Geometry: final body of the model. Coordinates: model frame, mm. A direction names the side the tool comes from. Give positions to 0.01 mm unless a question says otherwise; leave off trailing zeros. Order: outer loops, then holes, each group sorted by start corner. A loop starts at its lowest first (then second) coordinate and runs counter-clockwise, first axis right, second up. Notation, with made-up numbers: M 13,63.5 L 38,63.5 A30 ccw 38,91.5 Z; hole C 89.5,-5 d7. An arc over 180 degrees is marked long. Use CSV: the item, a comma, the result in double quotes.
```python
from build123d import *

# Parameters (mm, degrees)
BOSS_EXTRUDE2_DEPTH  = 4
SKETCH2_W            = 390
SKETCH2_H            = 480
BOSS_EXTRUDE3_DEPTH  = 4
SKETCH3_W            = 380
SKETCH3_H            = 470
BOSS_EXTRUDE4_DEPTH  = 4
SKETCH4_W            = 370
SKETCH4_H            = 460
BOSS_EXTRUDE5_DEPTH  = 4
SKETCH5_W            = 360
SKETCH5_H            = 450
BOSS_EXTRUDE6_DEPTH  = 4
SKETCH6_W            = 280
SKETCH6_H            = 370
CUT_EXTRUDE1_DEPTH   = 4
SKETCH7_W            = 270
SKETCH7_H            = 360
CUT_EXTRUDE2_DEPTH   = 4
SKETCH8_W            = 260
SKETCH8_H            = 350
CUT_EXTRUDE3_DEPTH   = 4
SKETCH9_W            = 250
SKETCH9_H            = 340
CUT_EXTRUDE4_DEPTH   = 4
SKETCH11_W           = 190
SKETCH11_H           = 280
BOSS_EXTRUDE7_DEPTH  = 4
SKETCH12_W           = 180
SKETCH12_H           = 270
BOSS_EXTRUDE8_DEPTH  = 4
SKETCH13_W           = 170
SKETCH13_H           = 260
BOSS_EXTRUDE9_DEPTH  = 4
SKETCH14_W           = 160
SKETCH14_H           = 250
BOSS_EXTRUDE10_DEPTH = 4
SKETCH15_W           = 20
SKETCH15_H           = 20
BOSS_EXTRUDE11_DEPTH = 5
SKETCH16_W           = 15
SKETCH16_H           = 15
BOSS_EXTRUDE12_DEPTH = 5
SKETCH17_W           = 10
SKETCH17_H           = 10
BOSS_EXTRUDE13_DEPTH = 20
BOSS_EXTRUDE14_REACH = 302
SKETCH18_W           = 10
SKETCH18_H           = 10
SKETCH19_W           = 35
SKETCH19_H           = 50
CUT_EXTRUDE5_DEPTH   = 3


with BuildPart() as part:
    # Sketch1 → Boss-Extrude2 (new body)
    with BuildSketch(Plane.XY):
        Polygon((200, 0), (200, -20), (200, -245), (-200, -245), (-200, -20), (-200, 0), (-200, 245), (200, 245), align=None)
    extrude(amount=BOSS_EXTRUDE2_DEPTH)

    # Sketch2 → Boss-Extrude3 (add)
    with BuildSketch(Plane.XY.offset(4)):
        Rectangle(SKETCH2_W, SKETCH2_H)
    extrude(amount=BOSS_EXTRUDE3_DEPTH)

    # Sketch3 → Boss-Extrude4 (add)
    with BuildSketch(Plane.XY.offset(8)):
        Rectangle(SKETCH3_W, SKETCH3_H)
    extrude(amount=BOSS_EXTRUDE4_DEPTH)

    # Sketch4 → Boss-Extrude5 (add)
    with BuildSketch(Plane.XY.offset(12)):
        Rectangle(SKETCH4_W, SKETCH4_H)
    extrude(amount=BOSS_EXTRUDE5_DEPTH)

    # Sketch5 → Boss-Extrude6 (add)
    with BuildSketch(Plane.XY.offset(16)):
        Rectangle(SKETCH5_W, SKETCH5_H)
    extrude(amount=BOSS_EXTRUDE6_DEPTH)

    # Sketch6 → Cut-Extrude1 (cut)
    with BuildSketch(Plane.XY.offset(20)):
        Rectangle(SKETCH6_W, SKETCH6_H)
    extrude(amount=-CUT_EXTRUDE1_DEPTH, mode=Mode.SUBTRACT)

    # Sketch7 → Cut-Extrude2 (cut)
    with BuildSketch(Plane.XY.offset(16)):
        Rectangle(SKETCH7_W, SKETCH7_H)
    extrude(amount=-CUT_EXTRUDE2_DEPTH, mode=Mode.SUBTRACT)

    # Sketch8 → Cut-Extrude3 (cut)
    with BuildSketch(Plane.XY.offset(12)):
        Rectangle(SKETCH8_W, SKETCH8_H)
    extrude(amount=-CUT_EXTRUDE3_DEPTH, mode=Mode.SUBTRACT)

    # Sketch9 → Cut-Extrude4 (cut)
    with BuildSketch(Plane.XY.offset(8)):
        Rectangle(SKETCH9_W, SKETCH9_H)
    extrude(amount=-CUT_EXTRUDE4_DEPTH, mode=Mode.SUBTRACT)

    # Sketch11 → Boss-Extrude7 (add)
    with BuildSketch(Plane.XY.offset(4)):
        Rectangle(SKETCH11_W, SKETCH11_H)
    extrude(amount=BOSS_EXTRUDE7_DEPTH)

    # Sketch12 → Boss-Extrude8 (add)
    with BuildSketch(Plane.XY.offset(8)):
        Rectangle(SKETCH12_W, SKETCH12_H)
    extrude(amount=BOSS_EXTRUDE8_DEPTH)

    # Sketch13 → Boss-Extrude9 (add)
    with BuildSketch(Plane.XY.offset(12)):
        Rectangle(SKETCH13_W, SKETCH13_H)
    extrude(amount=BOSS_EXTRUDE9_DEPTH)

    # Sketch14 → Boss-Extrude10 (add)
    with BuildSketch(Plane.XY.offset(16)):
        Rectangle(SKETCH14_W, SKETCH14_H)
    extrude(amount=BOSS_EXTRUDE10_DEPTH)

    # Sketch15 → Boss-Extrude11 (add)
    with BuildSketch(Plane.XY.offset(20)):
        with Locations((160, 60)):
            Rectangle(SKETCH15_W, SKETCH15_H)
        with Locations((160, -60)):
            Rectangle(SKETCH15_W, SKETCH15_H)
    extrude(amount=BOSS_EXTRUDE11_DEPTH)

    # Sketch16 → Boss-Extrude12 (add)
    with BuildSketch(Plane.XY.offset(25)):
        with Locations((160, 60)):
            Rectangle(SKETCH16_W, SKETCH16_H)
        with Locations((160, -60)):
            Rectangle(SKETCH16_W, SKETCH16_H)
    extrude(amount=BOSS_EXTRUDE12_DEPTH)

    # Sketch17 → Boss-Extrude13 (add)
    with BuildSketch(Plane.XY.offset(30)):
        with Locations((160, 60)):
            Rectangle(SKETCH17_W, SKETCH17_H)
        with Locations((160, -60)):
            Rectangle(SKETCH17_W, SKETCH17_H)
    extrude(amount=BOSS_EXTRUDE13_DEPTH)

    # Sketch18 → Boss-Extrude14 (add, up to next)
    with BuildSketch(Plane.XZ.offset(-55), mode=Mode.PRIVATE) as boss_extrude14_sk1:
        with Locations((160, 45)):
            Rectangle(SKETCH18_W, SKETCH18_H)
    boss_extrude14_tool1 = extrude(boss_extrude14_sk1.sketch, amount=BOSS_EXTRUDE14_REACH, mode=Mode.PRIVATE) - part.part
    add(boss_extrude14_tool1.solids().sort_by_distance((160, 55, 45))[0])

    # Sketch19 → Cut-Extrude5 (cut)
    with BuildSketch(Plane(origin=(0, 0, 0), x_dir=(-1, 0, 0), z_dir=(0, 0, -1))):
        with Locations((182.5, 125)):
            Rectangle(SKETCH19_W, SKETCH19_H)
        with Locations((182.5, -175)):
            Rectangle(SKETCH19_W, SKETCH19_H)
    extrude(amount=-CUT_EXTRUDE5_DEPTH, mode=Mode.SUBTRACT)


solid = part.part
```
1. Pin query (flat end, axial travel): pin 1 Ø10 at (x, z) = (19.5, 11) entering from -Y; pin 2 Ø1 at (x, z) = (24, 15) entering from +Y; pin 3 Ø1 at (y, z) = (60.5, 24) entering from -X. Return the tip coordinate at first contact, or that it passes through.
Answer:
pin 1,"y = -240"
pin 2,"y = 230"
pin 3,"x = 150"
2. Section A-A, the plane x = -172. Return the cut outline in (y, z), plus the area to 3 significant figures.
Answer:
outline,"M -245,0 L -200,0 L -200,3 L -150,3 L -150,0 L 100,0 L 100,3 L 150,3 L 150,0 L 245,0 L 245,4 L 240,4 L 240,8 L 235,8 L 235,12 L 230,12 L 230,16 L 225,16 L 225,20 L -225,20 L -225,16 L -230,16 L -230,12 L -235,12 L -235,8 L -240,8 L -240,4 L -245,4 Z"
area,"9,100 mm2"
3. Pull-direction query (Z, two-part tool) for faces 1 (the face through (169, -60, 25)), 2 (the face through (-1, 2, 20)), 3 (the face through (-182, -175, 3)), 4 (the face through (160, 65, 40)); classes: +Z half, -Z half, draft (parallel to the pull), parting line (faces both ways), or undercut.
Answer:
face 1,"undercut"
face 2,"+Z half"
face 3,"-Z half"
face 4,"draft"
4. Line query: line 1 (Y direction, x = 16, z = 19.5); line 2 (X direction, y = 40.5, z = 4.5); line 3 (Y direction, x = 104, z = 7). Output: solid intervals per line, ascending.
Answer:
line 1,"-225 to -185, -125 to 125, 185 to 225"
line 2,"-195 to -125, -95 to 95, 125 to 195"
line 3,"-240 to -170, 170 to 240"
5. Reachability of faces 5 (the face through (165, 1, 44)), 6 (the face through (160, 1, 50)), 7 (the face through (-131, 1, 12)), 8 (the face through (-182, 125, 3)), 9 (the face through (160, 1, 40)) from +Z, -Z, +X, -X, +Y, -Y: full face, straight path, thin tool, end or side. Return the list, or none.
Answer:
face 5,"+Z, +X, +Y, -Y"
face 6,"+Z, +X, -X, +Y, -Y"
face 7,"+Z"
face 8,"-Z, -X"
face 9,"+X, -X"
